Verification items for the finished model (mm, model axes). Face numbers are marked on the shaded views. Round coordinates to 2 decimals unless told otherwise and drop trailing zeros. Order: outer loops, then holes, each group sorted by start corner. A loop starts at its lowest first (then second) coordinate and runs counter-clockwise, first axis right, second up. Notation, with made-up numbers: (-5.75, 24) -> (21.25, 24) arc R22 cw to (21.25, 60) -> close; hole circle Ø3 at (80.25, -19.5). An arc over 180 degrees is marked (long way). Return JSON: item names as keys, results as strings. Group by question number.
1) Section check C-C on z = -0.75. Enter the section's corners in (x, y).
2) Section check B-B on x = 0. Enter the section's corners in (y, z), plus the area to 3 significant figures.
3) Section check D-D on x = -14. Enter the section's corners in (y, z), plus the area to 3 significant figures.
4) Draft check along Y on the marked faces 1, 2 and 3. Enter one of: pulls with the +Y half, pulls with the -Y half, needs draft (parallel to the pull), parting line crosses it, or undercut.
5) Scan lines: L1, parallel to Y at x = 12.5, z = 1; L2, parallel to Y at x = 0, z = -2.5; L3, parallel to X at y = 1, z = -4.5. Record each from-to range of solid material in increasing order.
6) Depth check by flat-ended pin: pin 1 (5 mm diameter, centred on x = -2, z = 1, fed in from -Y); pin 2 (6 mm diameter, centred on x = 18.5, z = 0.5, fed in from -Y); pin 3 (4 mm diameter, centred on x = 25, y = 0, fed in from +Z); pin 4 (2 mm diameter, centred on x = 17.5, z = -3, fed in from +Y). Enter the tip coordinate at first touch or a pass-through.
7) Section check A-A on y = 0. Enter the section's corners in (x, z), plus the area to 3 significant figures.
```python
from build123d import *

# Parameters (mm, degrees)
ESBO_O2_W                = 80
ESBO_O2_H                = 117.2
RESSALTO_EXTRUS_O2_DEPTH = 5
ESBO_O3_R                = 3
CORTE_EXTRUS_O1_DEPTH    = 11
ESBO_O4_R                = 3.3
CORTE_EXTRUS_O2_DEPTH    = 34.5
PADR_OCIRCULAR1_COUNT    = 6
ESBO_O12_W               = 80
ESBO_O12_H               = 17.2
CORTE_EXTRUS_O7_DEPTH    = 11
ESBO_O13_W               = 80
ESBO_O13_H               = 100
ESBO_O13_R               = 31
CORTE_EXTRUS_O8_DEPTH    = 11


with BuildPart() as part:
    # Esboço2 → Ressalto-extrusão2 (new body, symmetric)
    with BuildSketch(Plane.XY):
        Rectangle(ESBO_O2_W, ESBO_O2_H)
    extrude(amount=RESSALTO_EXTRUS_O2_DEPTH, both=True)

    # Esboço3 → Corte-extrusão1 (cut, through all)
    with BuildSketch(Plane.XY.offset(5)):
        Circle(ESBO_O3_R)
    extrude(amount=-CORTE_EXTRUS_O1_DEPTH, mode=Mode.SUBTRACT)

    # Esboço4 → Corte-extrusão2 (cut)
    with BuildSketch(Plane.XY.offset(5)):
        with Locations((12.5, 21.650635095)):
            Circle(ESBO_O4_R)
    corte_extrus_o2 = extrude(amount=-CORTE_EXTRUS_O2_DEPTH, mode=Mode.SUBTRACT)

    # PadrãoCircular1: Corte-extrusão2 ×6 about axis
    padr_ocircular1_axis = Axis((0, 0, 0), (0, 0, 1))
    for i in range(1, PADR_OCIRCULAR1_COUNT):
        add(corte_extrus_o2.rotate(padr_ocircular1_axis, i * 360 / PADR_OCIRCULAR1_COUNT), mode=Mode.SUBTRACT)

    # Esboço12 → Corte-extrusão7 (cut, through all)
    with BuildSketch(Plane.XY.offset(5)):
        with Locations((0, -50)):
            Rectangle(ESBO_O12_W, ESBO_O12_H)
    extrude(amount=-CORTE_EXTRUS_O7_DEPTH, mode=Mode.SUBTRACT)

    # Esboço13 → Corte-extrusão8 (cut, through all)
    with BuildSketch(Plane.XY.offset(5)):
        with Locations((0, 8.6)):
            Rectangle(ESBO_O13_W, ESBO_O13_H)
        Circle(ESBO_O13_R, mode=Mode.SUBTRACT)
    extrude(amount=-CORTE_EXTRUS_O8_DEPTH, mode=Mode.SUBTRACT)


solid = part.part
```
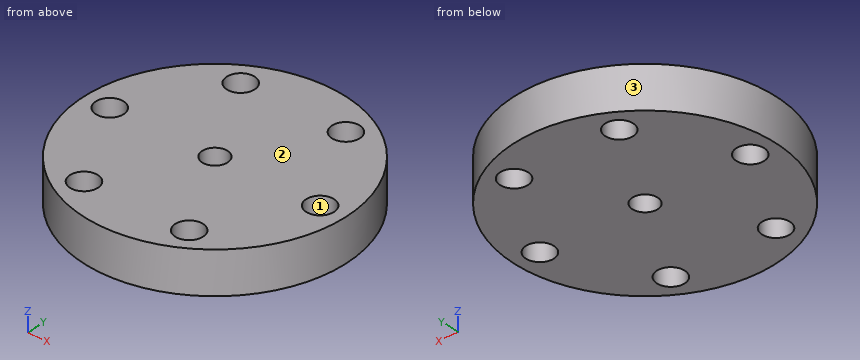
Check result:
{
 "1": {"outline": "circle Ø62 at (0, 0); hole circle Ø6.6 at (-25, 0); hole circle Ø6.6 at (-12.5, -21.65); hole circle Ø6.6 at (-12.5, 21.65); hole circle Ø6 at (0, 0); hole circle Ø6.6 at (12.5, -21.65); hole circle Ø6.6 at (12.5, 21.65); hole circle Ø6.6 at (25, 0)"},
 "2": {"outline": "(-31, -5) -> (-3, -5) -> (-3, 5) -> (-31, 5) -> close; (3, -5) -> (31, -5) -> (31, 5) -> (3, 5) -> close", "area": "560 mm^2"},
 "3": {"outline": "(-27.66, -5) -> (-24.59, -5) -> (-24.59, 5) -> (-27.66, 5) -> close; (-18.71, -5) -> (18.71, -5) -> (18.71, 5) -> (-18.71, 5) -> close; (24.59, -5) -> (27.66, -5) -> (27.66, 5) -> (24.59, 5) -> close", "area": "436 mm^2"},
 "4": {"face 1": "undercut", "face 2": "needs draft", "face 3": "parting line crosses it"},
 "5": {"L1": "-28.37 to -24.95, -18.35 to 18.35, 24.95 to 28.37", "L2": "-31 to -3, 3 to 31", "L3": "-30.98 to -28.14, -21.86 to -2.83, 2.83 to 21.86, 28.14 to 30.98"},
 "6": {"pin 1": "y = -31", "pin 2": "y = -26.85", "pin 3": "through", "pin 4": "y = 26.24"},
 "7": {"outline": "(-31, -5) -> (-28.3, -5) -> (-28.3, 5) -> (-31, 5) -> close; (-21.7, -5) -> (-3, -5) -> (-3, 5) -> (-21.7, 5) -> close; (3, -5) -> (21.7, -5) -> (21.7, 5) -> (3, 5) -> close; (28.3, -5) -> (31, -5) -> (31, 5) -> (28.3, 5) -> close", "area": "428 mm^2"}
}
